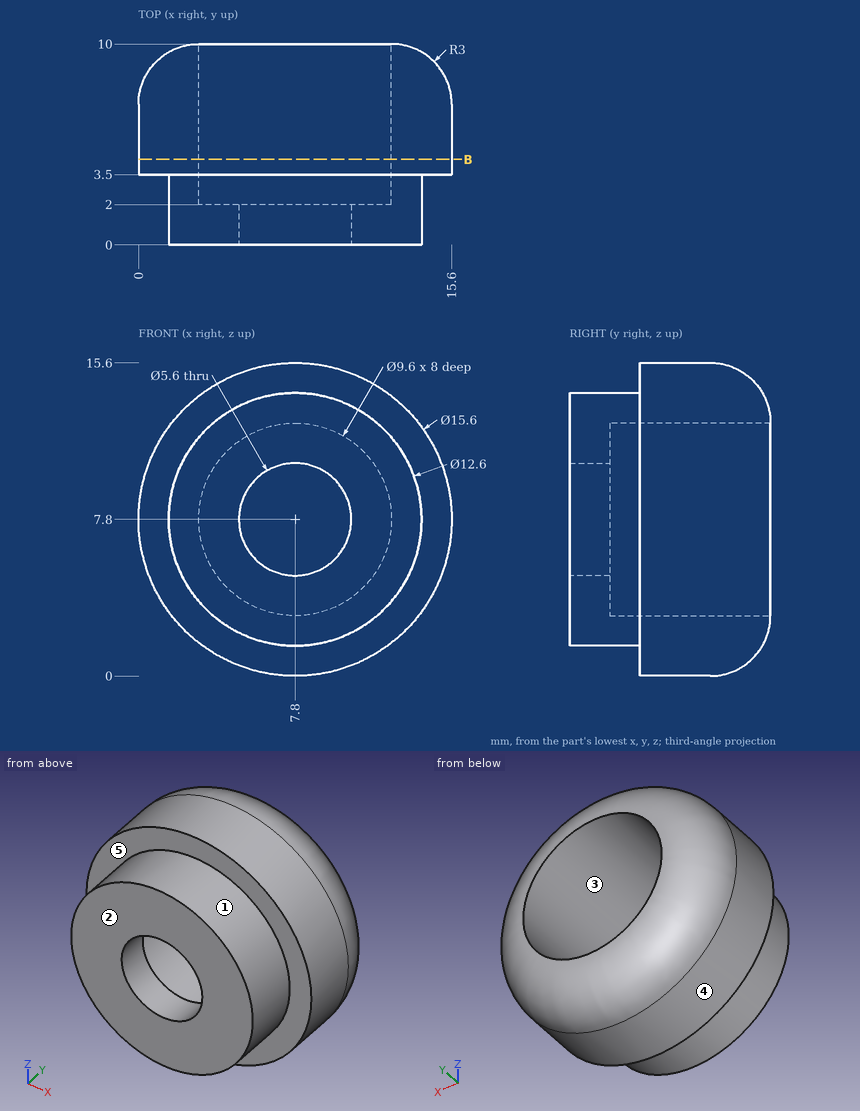
Design review of the part shown in the three views and the two pictorial views. Dimensions are in mm from the part's minimum x, y and z. A direction names the side the tool comes from. Coordinates: 2 decimals unless noted, no trailing zeros. Order: outer loops, then holes, each group sorted by start corner. A loop starts at its lowest first (then second) coordinate and runs counter-clockwise, first axis right, second up. Notation, with made-up numbers: (43, 58) - (61, 58) arc R17 cw to (61, 69) - close; hole circle Ø9 at (79.5, 89.25). An arc over 180 degrees is marked (long way). Answer as CSV lines item,"result". Start each with the question number.
1) Add section B-B (y = 4.25). State the section outline as (x, z) points.
2) Draft analysis for pull direction X (two halves, no side actions). For the marked faces 1, 2 and 3, state which applies: +X half, -X half, draft (parallel to the pull), parting line (faces both ways), or undercut.
3) To check wall thickness, follow line 1 along X through (y, z) = (1.5, 7.8); line 2 along Y through (x, z) = (11.75, 8). State the ranges of each line that lie inside material, in increasing order. Write a range as [from, to].
4) Insertion check: P1, Ø5, axis at x = 9.5, z = 8, coming from the +Y side; P2, Ø1, axis at y = 6.5, z = 5, coming from the -X side; P3, Ø2, axis at y = 3.5, z = 14, coming from the +X side; P4, Ø4.5, axis at x = 7.8, z = 7.8, coming from the +Y side. Each pin has a flat end and moves straight along its axis. Give the tip position at first contact, or say it passes through.
5) Machinability: for the marked faces 4 and 5, which of the approach directions +Z, -Z, +X, -X, +Y, -Y give a long, thin tool a straight path to every point of the face, cutting with its end or side? Answer none if there is none.
Result:
1,outline,"circle Ø15.6 at (7.8, 7.8); hole circle Ø9.6 at (7.8, 7.8)"
2,face 1,"parting line"
2,face 2,"draft"
2,face 3,"undercut"
3,line 1,"[1.5, 5], [10.6, 14.1]"
3,line 2,"[0, 2]"
4,P1,"y = 2"
4,P2,"x = 0.35"
4,P3,"x = 13.61"
4,P4,"through"
5,face 4,"+Y, -Y"
5,face 5,"-Y"
